Model file for the job. Use its own axes, mm. A direction names the side the tool comes from. Coordinates: 2 decimals unless noted, no trailing zeros. Order: outer loops, then holes, each group sorted by start corner. A loop starts at its lowest first (then second) coordinate and runs counter-clockwise, first axis right, second up. Notation, with made-up numbers: (54, 79) -> (64, 79) arc R19 ccw to (64, 90) -> close; hole circle Ø5 at (36, 89). An arc over 180 degrees is marked (long way). Return JSON: item names as keys, results as strings. Group by question number.
1) Which spindle directions (+Z, -Z, +X, -X, +Y, -Y) get a long thin tool onto all of the face, cutting with end or side? Do faces 1 (the flat face through (-6.7, 3.88, 1.01)), 2 (the flat face through (6, 0, 2)). Say none if no direction does.
2) Probe line 1 (Y direction, x = 0, z = 5); line 2 (Y direction, x = 2, z = 6.5); line 3 (Z direction, x = 11, y = -8). List the from-to ranges inside material, lowest first.
3) Cut at B-B (x = 0). Write the cut outline in (y, z).
4) Cut at A-A (y = 0). Write the cut outline in (x, z), and give its area (3 significant figures).
5) Flat gauge pins, fed straight in: pin 1 (1 mm diameter, centred on x = -4, y = 25, fed in from +Z); pin 2 (3 mm diameter, centred on x = -19.5, y = -23, fed in from +Z); pin 3 (1.6 mm diameter, centred on x = 14, z = 1.5, fed in from +Y). Where does each tip first touch, or does it go through?
6) Cut at C-C (y = 10.5). Write the cut outline in (x, z).
7) Cut at D-D (z = 3). Write the cut outline in (x, y).
8) Pull direction Y, two halves, no side cores. Call faces 3 (the flat face through (0, -7, 0)), 4 (the flat face through (-0.889, -15, 1)): +Y half, -Y half, draft (parallel to the pull), parting line (faces both ways), or undercut.
from build123d import *

# Parameters (mm, degrees)
F0_R      = 32.5
F1_DEPTH  = 10
F2_R      = 29.5
F3_DEPTH  = 8
F6_D      = 3.5
F8_DEPTH  = 2
F9_DEPTH  = 2
F10_DEPTH = 2
F11_DEPTH = 2
F4_R      = 3
F12_DEPTH = 10
F14_D     = 3.5


# Not quite as in the source:
# - the program builds the solid bodies; features that only make, move or delete a surface that nothing else refers to are left out


with BuildPart() as f1:
    # F0 (on Top) → F1 (new body)
    with BuildSketch(Plane.XY):
        Circle(F0_R)
    extrude(amount=F1_DEPTH)

    # F2 (on face) → F3 (cut)
    with BuildSketch(Plane.XY.offset(10)):
        Circle(F2_R)
    extrude(amount=-F3_DEPTH, mode=Mode.SUBTRACT)

    # F6 (through all)
    with Locations(Plane(origin=(0, 0, 0), x_dir=(1, 0, 0), z_dir=(0, 0, -1))):
        with Locations((0, 0)):
            Hole(F6_D / 2)

    # F7 (on face) → F8 (cut, through all)
    with BuildSketch(Plane.XY.offset(2)):
        Polygon((-7.741649435, 19.9890607288), (-16.1482516815, 16.9295235286), (-17.7019158656, 8.1194238235), (-10.8489778032, 2.3688613186), (-2.4423755567, 5.4283985188), (-0.8887113726, 14.2384982239), align=None)
    extrude(amount=-F8_DEPTH, mode=Mode.SUBTRACT)

    # F7 (on face) → F9 (cut, through all)
    with BuildSketch(Plane.XY.offset(2)):
        Polygon((-0.8887113726, -11.5674306203), (-0.8887113726, -18.4087138127), (5.0360136665, -21.8293554089), (10.9607387056, -18.4087138127), (10.9607387056, -11.5674306203), (5.0360136665, -8.1467890241), align=None)
    extrude(amount=-F9_DEPTH, mode=Mode.SUBTRACT)

    # F7 (on face) → F10 (cut, through all)
    with BuildSketch(Plane.XY.offset(2)):
        Polygon((-13.7885178521, -13.7792561938), (-10.1013832644, -10.1707357179), (-10.6237473641, -5.0381421005), (-14.9622593298, -2.2464230215), (-19.8499311619, -3.897799888), (-21.6062462804, -8.7487522375), (-18.9086635788, -13.1464140096), align=None)
    extrude(amount=-F10_DEPTH, mode=Mode.SUBTRACT)

    # F7 (on face) → F11 (cut, through all)
    with BuildSketch(Plane.XY.offset(2)):
        Polygon((11.8978734544, 5.9852199629), (17.9896090695, 5.9852199629), (21.0354768771, 11.2608177587), (17.9896090695, 16.5364155546), (11.8978734544, 16.5364155546), (8.8520056468, 11.2608177587), align=None)
    extrude(amount=-F11_DEPTH, mode=Mode.SUBTRACT)

    # F4 (on face) → F12 (join)
    with BuildSketch(Plane.XY.offset(2)):
        Circle(F4_R)
    extrude(amount=F12_DEPTH)

    # F14 (through all)
    with Locations(Plane.XY.offset(12)):
        with Locations((0, 0)):
            Hole(F14_D / 2)


solid = f1.part
Answers below:
{
 "1": {"face 1": "+Z, -Z", "face 2": "+Z"},
 "2": {"line 1": "y = -32.5 to -29.5, -3 to -1.75, 1.75 to 3, 29.5 to 32.5", "line 2": "y = -32.44 to -29.43, -2.24 to 2.24, 29.43 to 32.44", "line 3": "z = 0 to 2"},
 "3": {"outline": "(-32.5, 0) -> (-18.92, 0) -> (-18.92, 2) -> (-29.5, 2) -> (-29.5, 10) -> (-32.5, 10) -> close; (-11.05, 0) -> (-1.75, 0) -> (-1.75, 12) -> (-3, 12) -> (-3, 2) -> (-11.05, 2) -> close; (1.75, 0) -> (32.5, 0) -> (32.5, 10) -> (29.5, 10) -> (29.5, 2) -> (3, 2) -> (3, 12) -> (1.75, 12) -> close"},
 "4": {"outline": "(-32.5, 0) -> (-1.75, 0) -> (-1.75, 12) -> (-3, 12) -> (-3, 2) -> (-29.5, 2) -> (-29.5, 10) -> (-32.5, 10) -> close; (1.75, 0) -> (32.5, 0) -> (32.5, 10) -> (29.5, 10) -> (29.5, 2) -> (3, 2) -> (3, 12) -> (1.75, 12) -> close", "area": "196 mm^2"},
 "5": {"pin 1": "stops at z = 2", "pin 2": "stops at z = 10", "pin 3": "stops at y = 29.7"},
 "6": {"outline": "(-30.76, 0) -> (-17.28, 0) -> (-17.28, 2) -> (-27.57, 2) -> (-27.57, 10) -> (-30.76, 10) -> close; (-1.55, 0) -> (9.29, 0) -> (9.29, 2) -> (-1.55, 2) -> close; (20.6, 0) -> (30.76, 0) -> (30.76, 10) -> (27.57, 10) -> (27.57, 2) -> (20.6, 2) -> close"},
 "7": {"outline": "circle Ø65 at (0, 0); circle Ø6 at (0, 0); hole circle Ø59 at (0, 0); hole circle Ø3.5 at (0, 0)"},
 "8": {"face 3": "draft", "face 4": "undercut"}
}
